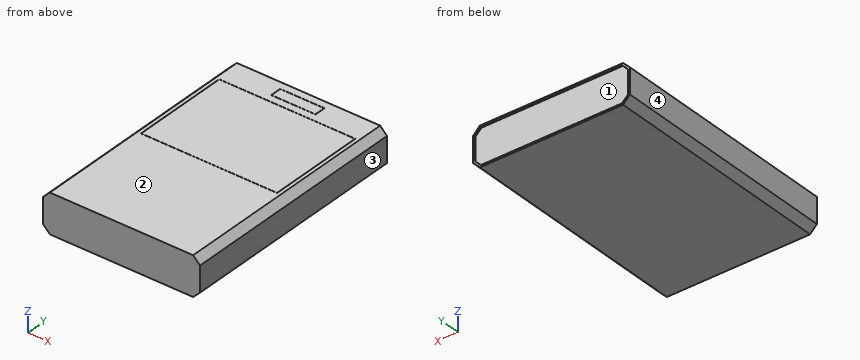
from build123d import *

# Parameters (mm, degrees)
SKETCH2_W           = 80
SKETCH2_H           = 120
BOSS_EXTRUDE1_DEPTH = 20
CHAMFER1_SIZE       = 3.5
CUT_EXTRUDE1_DEPTH  = 0.5
FILLET1_R           = 0.1
SKETCH4_W           = 22.384
SKETCH4_H           = 5.584
CUT_EXTRUDE2_DEPTH  = 0.1
SKETCH6_W           = 69.22
SKETCH6_H           = 50.02
CUT_EXTRUDE4_DEPTH  = 0.1


with BuildPart() as part:
    # Sketch2 → Boss-Extrude1 (new body)
    with BuildSketch(Plane.XY):
        Rectangle(SKETCH2_W, SKETCH2_H)
    extrude(amount=BOSS_EXTRUDE1_DEPTH)

    # Chamfer1
    chamfer1_edges = [part.edges().sort_by_distance(p)[0] for p in [
        (-40, 0, 20),
        (40, 0, 20),
        (-40, 0, 0),
        (40, 0, 0),
    ]]
    chamfer(chamfer1_edges, length=CHAMFER1_SIZE)

    # Sketch3 → Cut-Extrude1 (cut)
    with BuildSketch(Plane(origin=(0, 60, 0), x_dir=(1, 0, 0), z_dir=(0, 1, 0))):
        Polygon((-36, -19), (36, -19), (39, -16), (39, -4), (36, -1), (-36, -1), (-39, -4), (-39, -16), align=None)
    extrude(amount=-CUT_EXTRUDE1_DEPTH, mode=Mode.SUBTRACT)

    # Fillet1
    fillet1_edges = [part.edges().sort_by_distance(p)[0] for p in [
        (-40, 0, 16.5),
        (-40, 0, 3.5),
        (0, 60, 0),
        (36.5, 0, 0),
        (-36.5, 0, 0),
        (0, 60, 20),
        (40, 60, 10),
        (38.25, 60, 1.75),
        (38.25, 60, 18.25),
        (-38.25, 60, 18.25),
        (-38.25, 60, 1.75),
        (36.5, 0, 20),
        (-36.5, 0, 20),
        (40, 0, 3.5),
        (40, 0, 16.5),
        (-37.5, 60, 2.5),
        (-39, 59.75, 4),
        (0, 60, 1),
        (-36, 59.75, 1),
        (37.5, 60, 2.5),
        (36, 59.75, 1),
        (39, 59.75, 4),
        (39, 59.75, 16),
        (36, 59.75, 19),
        (-36, 59.75, 19),
        (-39, 60, 10),
        (-39, 59.75, 16),
        (-37.5, 60, 17.5),
        (0, 60, 19),
        (37.5, 60, 17.5),
        (39, 60, 10),
    ]]
    fillet(fillet1_edges, radius=FILLET1_R)

    # Sketch4 → Cut-Extrude2 (cut)
    with BuildSketch(Plane.XY.offset(20)):
        with BuildLine():
            Line((-11.192, 50.208), (11.192, 50.208))
            ThreePointArc((11.192, 50.208), (11.262710678, 50.237289322), (11.292, 50.308))
            Line((11.292, 50.308), (11.292, 55.892))
            ThreePointArc((11.292, 55.892), (11.262710678, 55.962710678), (11.192, 55.992))
            Line((11.192, 55.992), (-11.192, 55.992))
            ThreePointArc((-11.192, 55.992), (-11.262710678, 55.962710678), (-11.292, 55.892))
            Line((-11.292, 55.892), (-11.292, 50.308))
            ThreePointArc((-11.292, 50.308), (-11.262710678, 50.237289322), (-11.192, 50.208))
        make_face()
        with Locations((0, 53.1)):
            Rectangle(SKETCH4_W, SKETCH4_H, mode=Mode.SUBTRACT)
    extrude(amount=-CUT_EXTRUDE2_DEPTH, mode=Mode.SUBTRACT)

    # Sketch6 → Cut-Extrude4 (cut)
    with BuildSketch(Plane.XY.offset(20)):
        with BuildLine():
            ThreePointArc((-34.71, 46.218), (-34.680710678, 46.288710678), (-34.61, 46.318))
            Line((-34.61, 46.318), (34.61, 46.318))
            ThreePointArc((34.61, 46.318), (34.680710678, 46.288710678), (34.71, 46.218))
            Line((34.71, 46.218), (34.71, -3.802))
            ThreePointArc((34.71, -3.802), (34.680710678, -3.872710678), (34.61, -3.902))
            Line((34.61, -3.902), (-34.61, -3.902))
            ThreePointArc((-34.61, -3.902), (-34.680710678, -3.872710678), (-34.71, -3.802))
            Line((-34.71, -3.802), (-34.71, 46.218))
        make_face()
        with Locations((0, 21.208)):
            Rectangle(SKETCH6_W, SKETCH6_H, mode=Mode.SUBTRACT)
    extrude(amount=-CUT_EXTRUDE4_DEPTH, mode=Mode.SUBTRACT)


solid = part.part
The listing builds one solid part. Answer for the finished solid, in the listing's coordinates (mm). Face numbers are marked on the shaded views. Coordinates: 2 decimals unless noted, no trailing zeros. Loops run counter-clockwise (first coordinate to the right, second up) from the corner with the lowest first, then second, coordinate; pieces in that order, holes last.
1) Find section B-B on y = 27.5. Write down the section's boundary in (x, z).
2) Find the intervals of material crossed by L1, parallel to Y at x = 15.5, z = 4.25; L2, parallel to Z at x = 36.5, y = 0; L3, parallel to X at y = 52.5, z = 18, in increasing order.
3) Determine the mould class of the marked faces 1, 2, 3 and 4 for opening direction X: pulls with the +X half, pulls with the -X half, needs draft (parallel to the pull), parting line crosses it, or undercut.
4) Find section A-A on y = -24.5. Write down the section's boundary in (x, z).
5) Flat-ended cylindrical pins translate along their axes: pin 1 Ø9 at (x, z) = (2, 10.5) entering from +Y; pin 2 Ø1 at (y, z) = (24.5, 2.5) entering from +X. Find the tip coordinate at first contact, or state that the pin passes through.
Values:
1. outline: (-40, 3.54) arc R0.1 ccw to (-39.97, 3.47) - (-36.53, 0.03) arc R0.1 ccw to (-36.46, 0) - (36.46, 0) arc R0.1 ccw to (36.53, 0.03) - (39.97, 3.47) arc R0.1 ccw to (40, 3.54) - (40, 16.46) arc R0.1 ccw to (39.97, 16.53) - (36.53, 19.97) arc R0.1 ccw to (36.46, 20) - (34.71, 20) - (34.71, 19.9) - (34.61, 19.9) - (34.61, 20) - (-34.61, 20) - (-34.61, 19.9) - (-34.71, 19.9) - (-34.71, 20) - (-36.46, 20) arc R0.1 ccw to (-36.53, 19.97) - (-39.97, 16.53) arc R0.1 ccw to (-40, 16.46) - close
2. L1: y = -60 to 59.5
2. L2: z = 0.01 to 19.99
2. L3: x = -38.5 to 38.5
3. face 1: undercut
3. face 2: needs draft
3. face 3: pulls with the +X half
3. face 4: pulls with the -X half
4. outline: (-40, 3.54) arc R0.1 ccw to (-39.97, 3.47) - (-36.53, 0.03) arc R0.1 ccw to (-36.46, 0) - (36.46, 0) arc R0.1 ccw to (36.53, 0.03) - (39.97, 3.47) arc R0.1 ccw to (40, 3.54) - (40, 16.46) arc R0.1 ccw to (39.97, 16.53) - (36.53, 19.97) arc R0.1 ccw to (36.46, 20) - (-36.46, 20) arc R0.1 ccw to (-36.53, 19.97) - (-39.97, 16.53) arc R0.1 ccw to (-40, 16.46) - close
5. pin 1: stops at y = 59.5
5. pin 2: stops at x = 39.5
